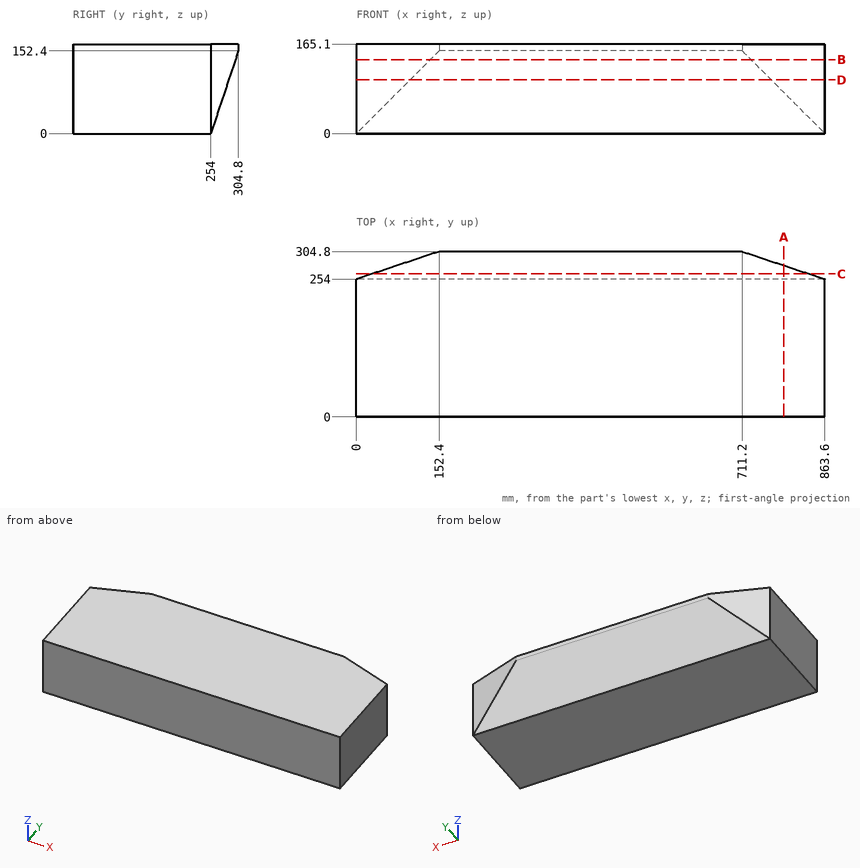
Job drawing, mm, ordinate dimensions from the low corner. One solid piece. Coordinates: 2 decimals unless noted, no trailing zeros. Order: outer loops, then holes, each group sorted by start corner. A loop starts at its lowest first (then second) coordinate and runs counter-clockwise, first axis right, second up. Notation, with made-up numbers: M 66.5,-6.5 L 93.5,-6.5 A32 ccw 93.5,29.5 Z; hole C 41,27.5 d8. An arc over 180 degrees is marked long. Answer as CSV lines item,"result".
(1) Band-saw the part on C-C, the plane y = 263.5. List the corners of the cut face in (x, z), then the cut area to 3 significant figures.
Geometry says:
outline,"M 28.5,28.5 L 835.1,28.5 L 835.1,165.1 L 28.5,165.1 Z"
area,"110,000 mm2"
(2) Flat gauge pins, fed straight in: pin 1 (10 mm diameter, centred on x = 296, z = 54, fed in from +Y); pin 2 (1.5 mm diameter, centred on x = 460.5, z = 125, fed in from +Y); pin 3 (1.5 mm diameter, centred on x = 736, z = 99.5, fed in from +Y); pin 4 (2 mm diameter, centred on x = 231, z = 115, fed in from -Y). Where does each tip first touch, or does it go through?
Geometry says:
pin 1,"stops at y = 273.67"
pin 2,"stops at y = 295.92"
pin 3,"stops at y = 287.42"
pin 4,"stops at y = 0"
(3) Band-saw the part on B-B, the plane z = 136.5. List the corners of the cut face in (x, y).
Geometry says:
outline,"M 0,0 L 863.6,0 L 863.6,254 L 727.1,299.5 L 136.5,299.5 L 0,254 Z"
(4) Wall check: line 1 along Y through (x, z) = (128.5, 10); line 2 along Y through (x, z) = (494, 34). Give the ranges that are in metal, low to high.
Geometry says:
line 1,"y = 0 to 257.33"
line 2,"y = 0 to 265.33"
(5) Band-saw the part on D-D, the plane z = 99. List the corners of the cut face in (x, y), then the cut area to 3 significant figures.
Geometry says:
outline,"M 0,0 L 863.6,0 L 863.6,254 L 764.6,287 L 99,287 L 0,254 Z"
area,"245,000 mm2"
(6) Band-saw the part on A-A, the plane x = 788. List the corners of the cut face in (y, z).
Geometry says:
outline,"M 0,0 L 254,0 L 279.2,75.6 L 279.2,165.1 L 0,165.1 Z"
